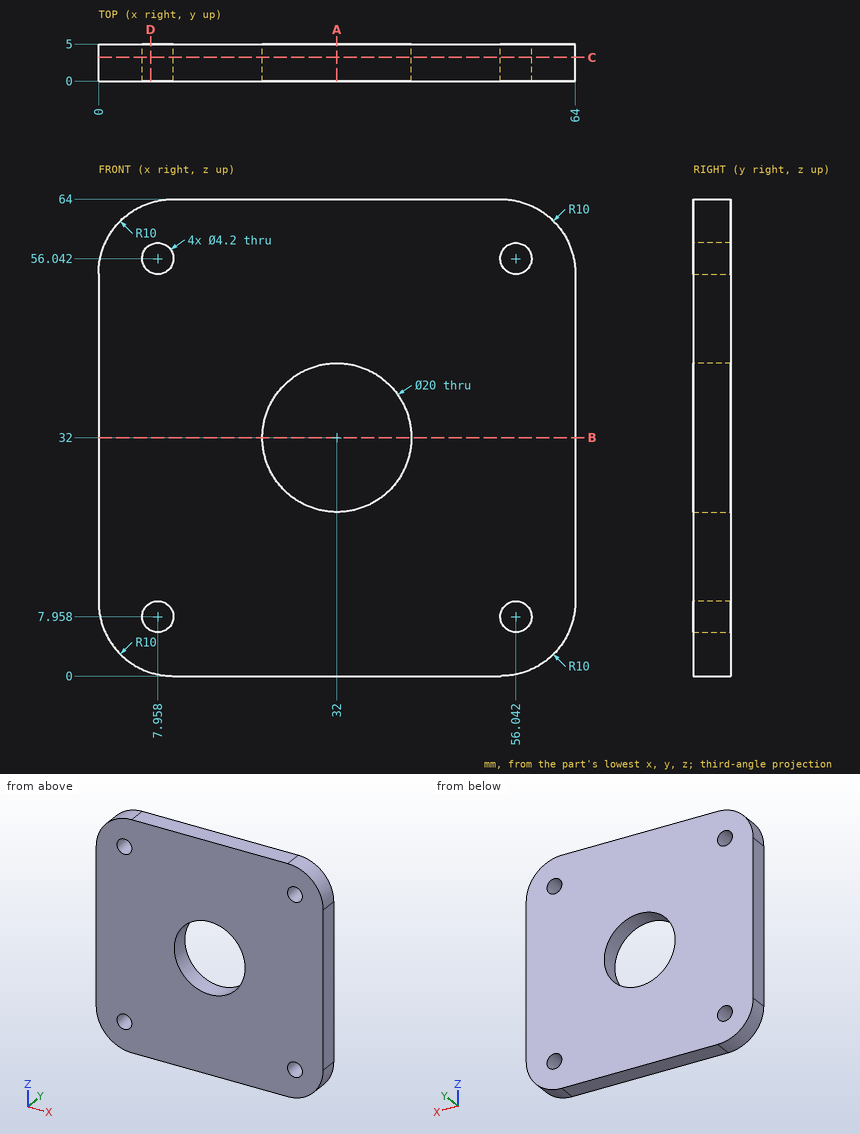
Can you work these out from the drawing? Everything is in mm from the part's minimum corner. Round coordinates to 2 decimals unless told otherwise and drop trailing zeros. Loops run counter-clockwise (first coordinate to the right, second up) from the corner with the lowest first, then second, coordinate; pieces in that order, holes last. Notation, with made-up numbers: M 13,30 L 35,30 A19 ccw 35,55 Z; hole C 56.5,15 d1. An arc over 180 degrees is marked long. Write item = value, one per line.
1. I want a section at B-B, the plane z = 32. Write out the boundary of the cut face in (x, y).
Results below:
outline = M 0,0 L 22,0 L 22,5 L 0,5 Z; M 42,0 L 64,0 L 64,5 L 42,5 Z
2. Will this pin go through, and if not, where does the flat tip stop? P1, Ø1.5, axis at y = 2.5, z = 55.5, coming from the -X side.
Results below:
P1 = 0.03
3. I want a section at A-A, the plane x = 32. Write out the boundary of the cut face in (y, z).
Results below:
outline = M 0,0 L 5,0 L 5,22 L 0,22 Z; M 0,42 L 5,42 L 5,64 L 0,64 Z
4. I want a section at D-D, the plane x = 7. Write out the boundary of the cut face in (y, z), and give its area (3 significant figures).
Results below:
outline = M 0,0.46 L 5,0.46 L 5,6.09 L 0,6.09 Z; M 0,9.83 L 5,9.83 L 5,54.17 L 0,54.17 Z; M 0,57.91 L 5,57.91 L 5,63.54 L 0,63.54 Z
area = 278 mm²
5. I want a section at C-C, the plane y = 3.2. Write out the boundary of the cut face in (x, z).
Results below:
outline = M 0,10 A10 ccw 10,0 L 54,0 A10 ccw 64,10 L 64,54 A10 ccw 54,64 L 10,64 A10 ccw 0,54 Z; hole C 7.96,7.96 d4.2; hole C 7.96,56.04 d4.2; hole C 32,32 d20; hole C 56.04,7.96 d4.2; hole C 56.04,56.04 d4.2
6. I need wall thicknesses on probe 1 along X at (y, z) = (0.3, 57); probe 2 along X at (y, z) = (1.75, 32); probe 3 along X at (y, z) = (3.9, 36) (1 decimal). Which ranges of each line are inside material? Lowest first, please.
Results below:
probe_1 = 0.46 to 6.09, 9.83 to 54.17, 57.91 to 63.54
probe_2 = 0 to 22, 42 to 64
probe_3 = 0 to 22.8, 41.2 to 64
